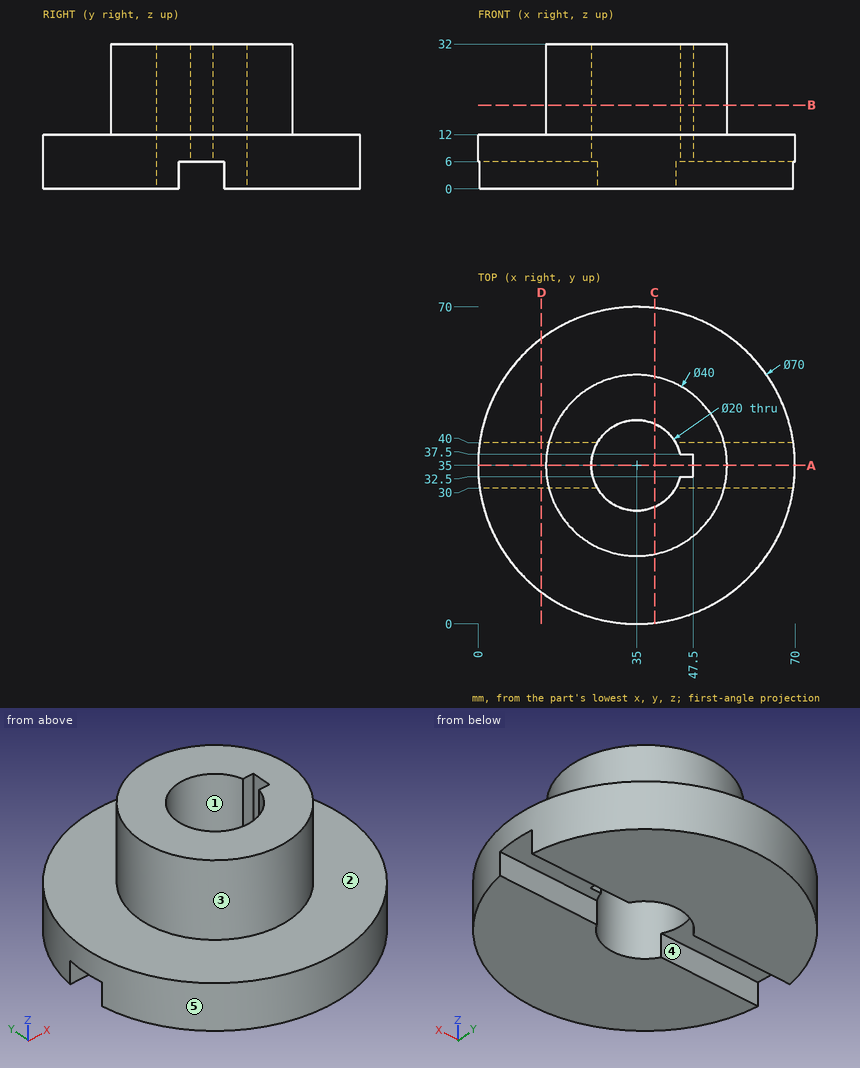
Answer from the drawing. Dimensions are ordinates in mm from the lowest x, y and z of the part. A direction names the side the tool comes from. Give positions to 0.01 mm unless a question says otherwise; leave off trailing zeros. Loops run counter-clockwise (first coordinate to the right, second up) from the corner with the lowest first, then second, coordinate; pieces in that order, holes last. Notation, with made-up numbers: (87.25, 4.5) -> (119.25, 4.5) arc R28 ccw to (119.25, 38.5) -> close; hole circle Ø4 at (80.25, 41.5). An arc over 180 degrees is marked (long way). Use a Markdown table: item, result.
Q1. Section C-C, the plane x = 39 is taken. Determine the outline of the cut face in (y, z).
Solved:
| item | result |
|---|---|
| outline | (0.23, 0) -> (25.83, 0) -> (25.83, 32) -> (15.4, 32) -> (15.4, 12) -> (0.23, 12) -> close; (44.17, 0) -> (69.77, 0) -> (69.77, 12) -> (54.6, 12) -> (54.6, 32) -> (44.17, 32) -> close |
Q2. Determine the mould class of the marked faces 1, 2 and 3 for opening direction Y: pulls with the +Y half, pulls with the -Y half, needs draft (parallel to the pull), parting line crosses it, or undercut.
Solved:
| item | result |
|---|---|
| face 1 | undercut |
| face 2 | needs draft |
| face 3 | parting line crosses it |
Q3. Section D-D, the plane x = 14 is taken. Determine the outline of the cut face in (y, z), then the cut area to 3 significant figures.
Solved:
| item | result |
|---|---|
| outline | (7, 0) -> (30, 0) -> (30, 6) -> (40, 6) -> (40, 0) -> (63, 0) -> (63, 12) -> (7, 12) -> close |
| area | 612 mm^2 |
Q4. Section A-A, the plane y = 35 is taken. Determine the outline of the cut face in (x, z).
Solved:
| item | result |
|---|---|
| outline | (0, 6) -> (25, 6) -> (25, 32) -> (15, 32) -> (15, 12) -> (0, 12) -> close; (47.5, 6) -> (70, 6) -> (70, 12) -> (55, 12) -> (55, 32) -> (47.5, 32) -> close |
Q5. Section B-B, the plane z = 18.5 is taken. Determine the outline of the cut face in (x, y), then the cut area to 3 significant figures.
Solved:
| item | result |
|---|---|
| outline | circle Ø40 at (35, 35); hole (44.68, 32.5) -> (47.5, 32.5) -> (47.5, 37.5) -> (44.68, 37.5) arc R10 ccw (long way) to start |
| area | 929 mm^2 |
Q6. Find the intervals of material crossed by line 1 along Y through (x, z) = (35, 22); line 2 along Z through (x, y) = (5, 32); line 3 along Z through (x, y) = (57, 9), in increasing order.
Solved:
| item | result |
|---|---|
| line 1 | y = 15 to 25, 45 to 55 |
| line 2 | z = 6 to 12 |
| line 3 | z = 0 to 12 |
Q7. Each of these flat-tipped pins is pushed along its axis until it touches: pin 1 (2.5 mm diameter, centred on y = 36, z = 12.5, fed in from -X); pin 2 (3 mm diameter, centred on y = 32.5, z = 22, fed in from +X) (3 decimals); pin 3 (12 mm diameter, centred on y = 13, z = 20.5, fed in from -X); pin 4 (3 mm diameter, centred on x = 46, z = 18, fed in from +Y). Where does it stop, or does it pass through?
Solved:
| item | result |
|---|---|
| pin 1 | stops at x = 0 |
| pin 2 | stops at x = 54.975 |
| pin 3 | stops at x = 23 |
| pin 4 | stops at y = 52.6 |
Q8. A tool of negligible diameter and unlimited length cuts with its end or side. For the marked faces 4 and 5, from which of +Z, -Z, +X, -X, +Y, -Y can it reach the whole face along a straight path? Write none if from no direction.
Solved:
| item | result |
|---|---|
| face 4 | -Z, +X, -X |
| face 5 | +Z, -Z |
